Part model, mm, in its own coordinate system. Face numbers are marked on the shaded views. A direction names the side the tool comes from. Round coordinates to 2 decimals unless told otherwise and drop trailing zeros. Write each loop counter-clockwise with the first axis right and the second up, starting at its lowest first coordinate (ties: lowest second). Pieces come first, ordered by that corner, then holes. Notation, with made-up numbers: M 88.5,76 L 141.5,76 A25 cw 141.5,113 Z; hole C 46,15.25 d5. An arc over 180 degrees is marked long. Use a Markdown table: item, result. Add a question column.
1) Slice it at B-B on x = -5.75. Write the cut outline in (y, z).
2) Two-plate mould, pull along Z, no slides. Class the marked faces 1, 2, 3 and 4: released by +Z, released by -Z, zero draft, split by the parting line, or undercut.
3) Wall check: probe 1 along X at (y, z) = (3.95, -8.75); probe 2 along X at (y, z) = (4.25, 2.5); probe 3 along Z at (x, y) = (5, 1.2). Give the ranges that are in metal, low to high.
4) Drop a flat-ended pin along its axis: P1, Ø2.5, axis at x = 4.75, z = 2.5, coming from the +Y side. Give the stop position or say it passes through.
5) Which spindle directions (+Z, -Z, +X, -X, +Y, -Y) get a long thin tool onto all of the face, cutting with end or side? Do the marked faces 5 and 6. Say none if no direction does.
6) Slice it at D-D on x = -0.5. Write the cut outline in (y, z).
7) Slice it at A-A on z = 2.5. Write the cut outline in (x, y).
8) Slice it at C-C on z = -8.75. Write the cut outline in (x, y), plus the area to 3 significant figures.
```python
from build123d import *

# Parameters (mm, degrees)
CROQUIS1_W              = 20
CROQUIS1_H              = 17.5
SALIENTE_EXTRUIR1_DEPTH = 8
CROQUIS1_4_W            = 20
CROQUIS1_4_H            = 7.5
SALIENTE_EXTRUIR2_DEPTH = 5
CROQUIS2_R              = 1.5
CORTAR_EXTRUIR1_DEPTH   = 5
CROQUIS3_R              = 1.5
CORTAR_EXTRUIR2_DEPTH   = 20
CROQUIS4_W              = 20
CROQUIS4_H              = 2
CORTAR_EXTRUIR3_DEPTH   = 35


with BuildPart() as part:
    # Croquis1 → Saliente-Extruir1 (new body)
    with BuildSketch(Plane(origin=(0, 0, 0), x_dir=(1, 0, 0), z_dir=(0, 1, 0))):
        with Locations((0, -3.75)):
            Rectangle(CROQUIS1_W, CROQUIS1_H)
    extrude(amount=SALIENTE_EXTRUIR1_DEPTH)

    # Croquis1<4> → Saliente-Extruir2 (add)
    with BuildSketch(Plane(origin=(0, 0, 0), x_dir=(1, 0, 0), z_dir=(0, 1, 0))):
        with Locations((0, 8.75)):
            Rectangle(CROQUIS1_4_W, CROQUIS1_4_H)
    extrude(amount=SALIENTE_EXTRUIR2_DEPTH)

    # Croquis2 → Cortar-Extruir1 (cut)
    with BuildSketch(Plane(origin=(0, 5, 0), x_dir=(1, 0, 0), z_dir=(0, 1, 0))):
        with Locations((-5, 8.75)):
            Circle(CROQUIS2_R)
        with Locations((5, 8.75)):
            Circle(CROQUIS2_R)
    extrude(amount=-CORTAR_EXTRUIR1_DEPTH, mode=Mode.SUBTRACT)

    # Croquis3 → Cortar-Extruir2 (cut)
    with BuildSketch(Plane(origin=(0, 8, 0), x_dir=(1, 0, 0), z_dir=(0, 1, 0))):
        with Locations((-4.75, -2.5)):
            Circle(CROQUIS3_R)
        with Locations((4.75, -2.5)):
            Circle(CROQUIS3_R)
    extrude(amount=-CORTAR_EXTRUIR2_DEPTH, mode=Mode.SUBTRACT)

    # Croquis4 → Cortar-Extruir3 (cut)
    with BuildSketch(Plane(origin=(0, 8, 0), x_dir=(1, 0, 0), z_dir=(0, 1, 0))):
        with Locations((0, -11.5)):
            Rectangle(CROQUIS4_W, CROQUIS4_H)
    extrude(amount=-CORTAR_EXTRUIR3_DEPTH, mode=Mode.SUBTRACT)


solid = part.part
```
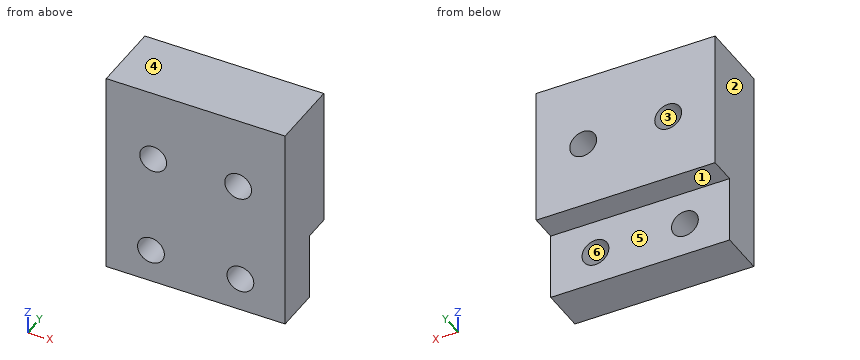
Entries:
| question | item | result |
|---|---|---|
| 1 | outline | M 0,-12.5 L 5,-12.5 L 5,-10.05 L 0,-10.05 Z; M 0,-7.45 L 5,-7.45 L 5,-5 L 8,-5 L 8,1.38 L 0,1.38 Z; M 0,3.62 L 8,3.62 L 8,10.5 L 0,10.5 Z |
| 2 | face 1 | released by -Z |
| 2 | face 2 | zero draft |
| 2 | face 3 | undercut |
| 2 | face 4 | released by +Z |
| 3 | probe 1 | x = -10 to -6.5, -3.5 to 3.5, 6.5 to 10 |
| 3 | probe 2 | x = -10 to -6.25, -3.25 to 3.25, 6.25 to 10 |
| 3 | probe 3 | z = -12.5 to -10.25, -7.25 to 1.02, 3.98 to 10.5 |
| 4 | P1 | passes through |
| 5 | face 5 | -Z, +X, -X, +Y |
| 5 | face 6 | +Y, -Y |
| 6 | outline | M 0,-12.5 L 5,-12.5 L 5,-5 L 8,-5 L 8,10.5 L 0,10.5 Z |
| 7 | outline | M -10,0 L -6.25,0 L -6.25,8 L -10,8 Z; M -3.25,0 L 3.25,0 L 3.25,8 L -3.25,8 Z; M 6.25,0 L 10,0 L 10,8 L 6.25,8 Z |
| 8 | outline | M -10,0 L -6.5,0 L -6.5,5 L -10,5 Z; M -3.5,0 L 3.5,0 L 3.5,5 L -3.5,5 Z; M 6.5,0 L 10,0 L 10,5 L 6.5,5 Z |
| 8 | area | 70.0 mm^2 |
